CAD build for the part. Positions are in the model's coordinates, mm. A direction names the side the tool comes from. Give positions to 0.01 mm unless a question says otherwise; leave off trailing zeros. Loops run counter-clockwise (first coordinate to the right, second up) from the corner with the lowest first, then second, coordinate; pieces in that order, holes last.
Item 1: Which spindle directions (+Z, -Z, +X, -X, +Y, -Y) get a long thin tool onto all of the face, cutting with end or side? Do faces 1 (the flat face through (29.46, -12.52, -23.64)), 2 (the flat face through (-15, -52, 4.762)). Say none if no direction does.
Item 2: Saw through at D-D on z = 11. Give the cut face in (x, y), plus the area to 3 significant figures.
Item 3: Mould opens along Z. For faces 3 (the cylindrical face through (41.922, 0.356, 0.558)), 4 (the flat face through (39, -25.4, 0)), 5 (the flat face through (30.832, -12.522, 23.502)) say: released by +Z, released by -Z, zero draft, split by the parting line, or undercut.
Item 4: Probe probe 1 along X at (y, z) = (-58.5, 1); probe 2 along Z at (x, y) = (54.61, 6); probe 3 along Y at (x, z) = (-5, 18.5). List the from-to ranges inside material, lowest first.
Item 5: Saw through at C-C on y = -11. Give the number of separate pieces and of enclosed holes in the cut face, plus the area to 3 significant figures.
Item 6: Drop flat-ended pins along their axis: P1, Ø3.5, axis at x = -15.5, y = -61, coming from the +Z side; P2, Ø10.5, axis at y = -49.5, z = 2, coming from the +X side (3 decimals); P3, Ø1.5, axis at y = -23.5, z = -11, coming from the +X side; P4, Ø10.5, axis at y = -58.5, z = 0, coming from the -X side (3 decimals). Give the stop position or say it passes through.
Item 7: Saw through at B-B on x = 0. Give the cut face in (y, z) (3 decimals).
from build123d import *

# Parameters (mm, degrees)
F0_R      = 12.7
F1_DEPTH  = 25.4
F2_DEPTH  = 52.324
F2_FACE_R = 28.575
F3_DEPTH  = 53.086
F4_DEPTH  = 25.4


with BuildPart() as f1:
    # F0 (on Front) → F1 (new body)
    with BuildSketch(Plane.XZ):
        with BuildLine():
            ThreePointArc((73.66, 0), (68.532063, 13.003025), (55.908961, 19.005662))
            ThreePointArc((55.908961, 19.005662), (35.573845, 0.726161), (54.457296, -19.049388))
            ThreePointArc((54.457296, -19.049388), (68.026287, -13.524265), (73.66, 0))
        make_face()
        with Locations((54.61, 0)):
            Circle(F0_R, mode=Mode.SUBTRACT)
        with BuildLine():
            ThreePointArc((5.16281, -28.104733), (21.955158, -18.289387), (28.575, 0))
            ThreePointArc((28.575, 0), (21.91626, 18.33598), (5.043369, 28.126412))
            ThreePointArc((5.043369, 28.126412), (-28.574936, -0.060696), (5.16281, -28.104733))
        make_face()
        with BuildLine():
            ThreePointArc((-11.773215, 4.7625), (0, 12.7), (11.773215, 4.7625))
            Line((11.773215, 4.7625), (19.05, 4.7625))
            Line((19.05, 4.7625), (19.05, -4.7625))
            Line((19.05, -4.7625), (11.773215, -4.7625))
            ThreePointArc((11.773215, -4.7625), (0, -12.7), (-11.773215, -4.7625))
            Line((-11.773215, -4.7625), (-19.05, -4.7625))
            Line((-19.05, -4.7625), (-19.05, 4.7625))
            Line((-19.05, 4.7625), (-11.773215, 4.7625))
        make_face(mode=Mode.SUBTRACT)
        with BuildLine():
            ThreePointArc((5.043369, 28.126412), (21.91626, 18.33598), (28.575, 0))
            ThreePointArc((28.575, 0), (21.955158, -18.289387), (5.16281, -28.104733))
            Line((5.16281, -28.104733), (54.457296, -19.049388))
            ThreePointArc((54.457296, -19.049388), (35.573845, 0.726161), (55.908961, 19.005662))
            Line((55.908961, 19.005662), (5.043369, 28.126412))
        make_face()
    extrude(amount=F1_DEPTH)

    # F0 (on Front) → F2 (join)
    with BuildSketch(Plane.XZ):
        with BuildLine():
            ThreePointArc((5.16281, -28.104733), (21.955158, -18.289387), (28.575, 0))
            ThreePointArc((28.575, 0), (21.91626, 18.33598), (5.043369, 28.126412))
            ThreePointArc((5.043369, 28.126412), (-28.574936, -0.060696), (5.16281, -28.104733))
        make_face()
        with BuildLine():
            ThreePointArc((-11.773215, 4.7625), (0, 12.7), (11.773215, 4.7625))
            Line((11.773215, 4.7625), (19.05, 4.7625))
            Line((19.05, 4.7625), (19.05, -4.7625))
            Line((19.05, -4.7625), (11.773215, -4.7625))
            ThreePointArc((11.773215, -4.7625), (0, -12.7), (-11.773215, -4.7625))
            Line((-11.773215, -4.7625), (-19.05, -4.7625))
            Line((-19.05, -4.7625), (-19.05, 4.7625))
            Line((-19.05, 4.7625), (-11.773215, 4.7625))
        make_face(mode=Mode.SUBTRACT)
    extrude(amount=F2_DEPTH)

    # F2_face (on face) → F3 (join)
    with BuildSketch(Plane.XZ.offset(52.324)):
        Circle(F2_FACE_R)
        with BuildLine():
            ThreePointArc((-11.773215, 4.7625), (0, 12.7), (11.773215, 4.7625))
            Line((11.773215, 4.7625), (19.05, 4.7625))
            Line((19.05, 4.7625), (19.05, -4.7625))
            Line((19.05, -4.7625), (11.773215, -4.7625))
            ThreePointArc((11.773215, -4.7625), (0, -12.7), (-11.773215, -4.7625))
            Line((-11.773215, -4.7625), (-19.05, -4.7625))
            Line((-19.05, -4.7625), (-19.05, 4.7625))
            Line((-19.05, 4.7625), (-11.773215, 4.7625))
        make_face(mode=Mode.SUBTRACT)
    extrude(amount=F3_DEPTH)

    # F0 (on Front) → F4 (join)
    with BuildSketch(Plane.XZ):
        with BuildLine():
            ThreePointArc((73.66, 0), (68.532063, 13.003025), (55.908961, 19.005662))
            ThreePointArc((55.908961, 19.005662), (35.573845, 0.726161), (54.457296, -19.049388))
            ThreePointArc((54.457296, -19.049388), (68.026287, -13.524265), (73.66, 0))
        make_face()
        with Locations((54.61, 0)):
            Circle(F0_R, mode=Mode.SUBTRACT)
    extrude(amount=-F4_DEPTH)


solid = f1.part
Results below:
1. face 1: -Z, +X, +Y, -Y
1. face 2: +Y, -Y
2. outline: (-26.37, -105.41) - (-6.35, -105.41) - (-6.35, 0) - (-26.37, 0) - close; (6.35, -105.41) - (26.37, -105.41) - (26.37, -25.4) - (48.26, -25.4) - (48.26, 25.4) - (39.06, 25.4) - (39.06, 0) - (6.35, 0) - close; (60.96, -25.4) - (70.16, -25.4) - (70.16, 25.4) - (60.96, 25.4) - close
2. area: 5,480 mm2
3. face 3: undercut
3. face 4: zero draft
3. face 5: released by +Z
4. probe 1: x = -28.56 to -19.05, 19.05 to 28.56
4. probe 2: z = -19.05 to -12.7, 12.7 to 19.05
4. probe 3: y = -105.41 to 0
5. separate pieces: 1
5. enclosed holes: 2
5. area: 3,340 mm2
6. P1: stops at z = 25.05
6. P2: stops at x = 28.575
6. P3: stops at x = 70.67
6. P4: stops at x = -28.575
7. outline: (-105.41, -28.575) - (0, -28.575) - (0, -12.7) - (-105.41, -12.7) - close; (-105.41, 12.7) - (0, 12.7) - (0, 28.575) - (-105.41, 28.575) - close
